Part print with two shaded views. Sizes in mm from the minimum x, y, z corner. Coordinates: 2 decimals unless noted, no trailing zeros. Loops run counter-clockwise (first coordinate to the right, second up) from the corner with the lowest first, then second, coordinate; pieces in that order, holes last.
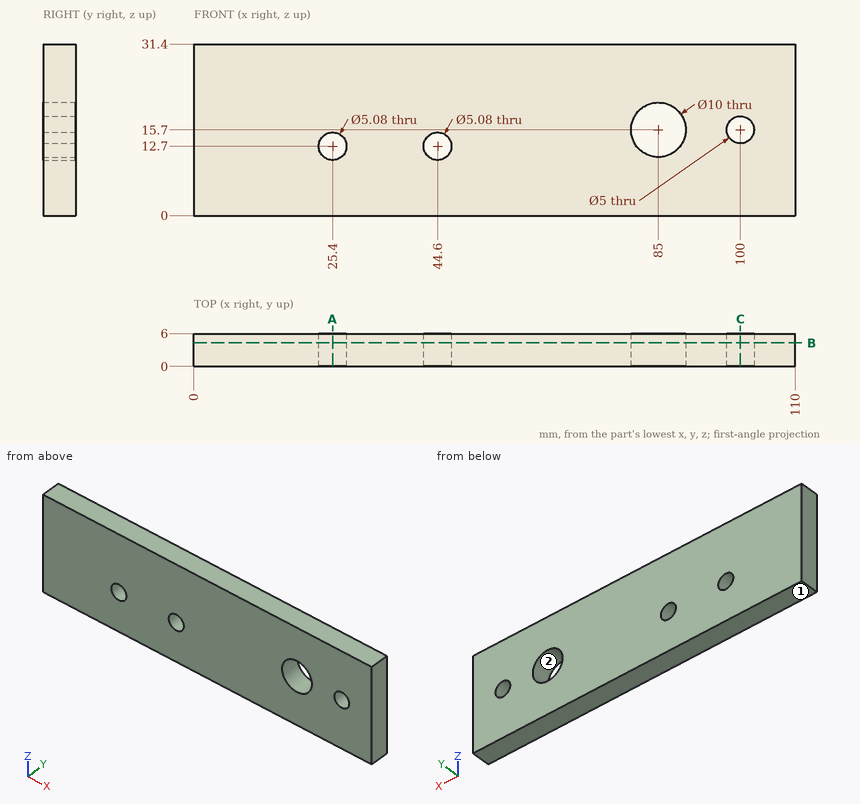
Q1. Drill centre lines: line 1 (X direction, y = 3.85, z = 15.7); line 2 (Z direction, x = 100, y = 3.5); line 3 (Z direction, x = 44.6, y = 1.8). Where is each one in solid material? Low to high.
Answers:
line 1: x = 0 to 80, 90 to 97.5, 102.5 to 110
line 2: z = 0 to 13.2, 18.2 to 31.4
line 3: z = 0 to 10.16, 15.24 to 31.4
Q2. Slice it at C-C (x = 100). List the corners of the cut face in (y, z).
Answers:
outline: (0, 0) - (6, 0) - (6, 13.2) - (0, 13.2) - close; (0, 18.2) - (6, 18.2) - (6, 31.4) - (0, 31.4) - close
Q3. Slice it at A-A (x = 25.4). List the corners of the cut face in (y, z).
Answers:
outline: (0, 0) - (6, 0) - (6, 10.16) - (0, 10.16) - close; (0, 15.24) - (6, 15.24) - (6, 31.4) - (0, 31.4) - close
Q4. Mould opens along X. For the marked faces 1 and 2 say: +X half, -X half, draft (parallel to the pull), parting line (faces both ways), or undercut.
Answers:
face 1: draft
face 2: undercut
Q5. Slice it at B-B (y = 4.3). List the corners of the cut face in (x, z).
Answers:
outline: (0, 0) - (110, 0) - (110, 31.4) - (0, 31.4) - close; hole circle Ø5.08 at (25.4, 12.7); hole circle Ø5.08 at (44.6, 12.7); hole circle Ø10 at (85, 15.7); hole circle Ø5 at (100, 15.7)
